Could you check a few things on this drawing? It's one solid part, dimensions in mm from its lowest x, y, z. A direction names the side the tool comes from. Round coordinates to 2 decimals unless told otherwise and drop trailing zeros. Loops run counter-clockwise (first coordinate to the right, second up) from the corner with the lowest first, then second, coordinate; pieces in that order, holes last. Notation, with made-up numbers: M 1.5,33 L 32.5,33 A7 cw 32.5,39 Z; hole C 20,15 d8. An arc over 180 degrees is marked long. Answer as CSV lines item,"result".
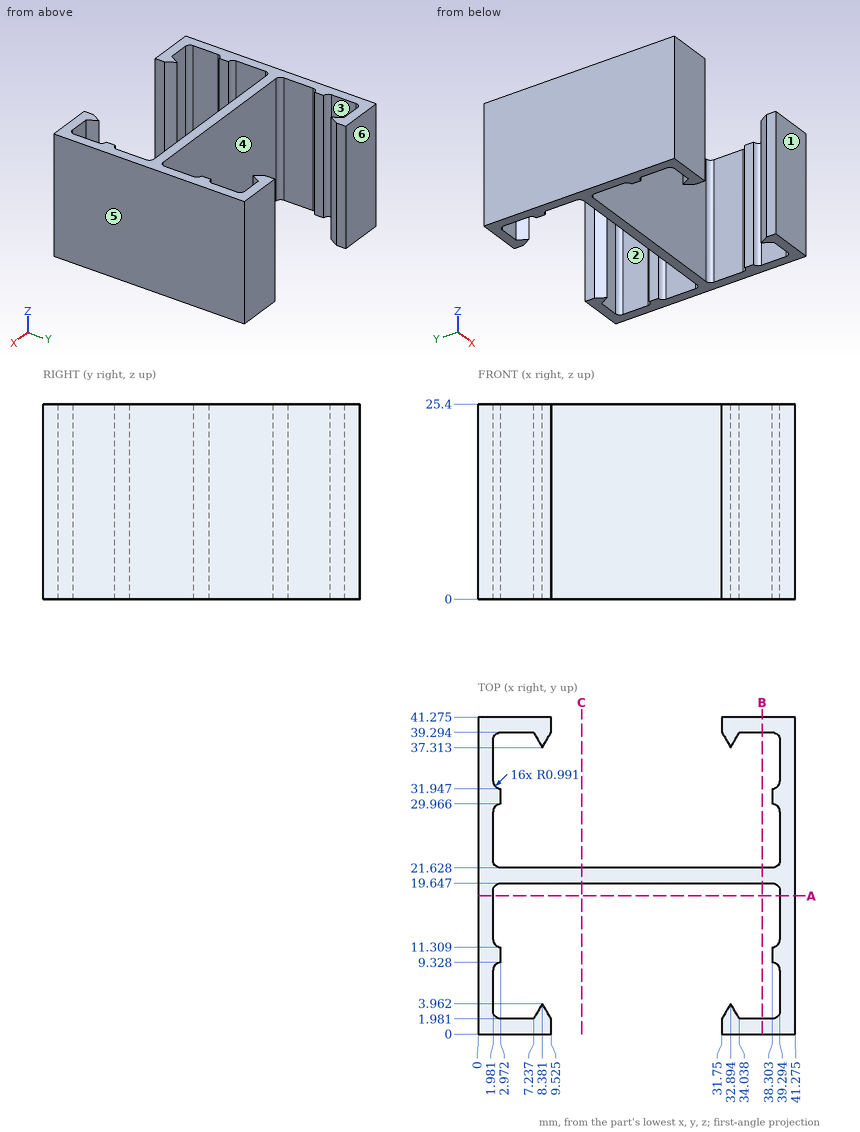
Item 1: If we section it at A-A on y = 18: Write out the boundary of the cut face in (x, z) (1 decimal).
Output:
outline,"M 0,0 L 2,0 L 2,25.4 L 0,25.4 Z; M 39.3,0 L 41.3,0 L 41.3,25.4 L 39.3,25.4 Z"
Item 2: On a 3-axis mill with a long thin cutter (end or side, diameter ignored), from which of +Z, -Z, +X, -X, +Y, -Y can I reach the whole of each face in a straight line? I mean the marked faces 1 and 2. Say none if no direction works.
Output:
face 1,"+Z, -Z, +X, -X, -Y"
face 2,"+Z, -Z"
Item 3: Will this pin go through, and if not, where does the flat tip stop? pin 1 (6 mm diameter, centred on x = 30.5, y = 20.5, fed in from -Z).
Output:
pin 1,"stops at z = 0"
Item 4: If we section it at C-C on x = 13.5: Write out the boundary of the cut face in (y, z).
Output:
outline,"M 19.65,0 L 21.63,0 L 21.63,25.4 L 19.65,25.4 Z"
Item 5: We'd pull the mould along Y, two halves only. Please class the marked faces 3, 4, 5 and 6: released by +Y, released by -Y, zero draft, split by the parting line, or undercut.
Output:
face 3,"undercut"
face 4,"undercut"
face 5,"zero draft"
face 6,"released by +Y"
Item 6: If we section it at B-B on x = 37: Write out the boundary of the cut face in (y, z) (1 decimal), then the cut area to 3 significant figures.
Output:
outline,"M 0,0 L 2,0 L 2,25.4 L 0,25.4 Z; M 19.6,0 L 21.6,0 L 21.6,25.4 L 19.6,25.4 Z; M 39.3,0 L 41.3,0 L 41.3,25.4 L 39.3,25.4 Z"
area,"151 mm2"
Item 7: If I drill on line 1 along X through (y, z) = (38, 11.25) (1 decimal); line 2 along X through (y, z) = (29, 14) (1 decimal); line 3 along Y through (x, z) = (17, 2.5), over which ranges is the centre line in solid material (lowest first)? Write a range as from..to.
Output:
line 1,"x = 0..2, 8..8.8, 32.5..33.3, 39.3..41.3"
line 2,"x = 0..2, 39.3..41.3"
line 3,"y = 19.65..21.63"
